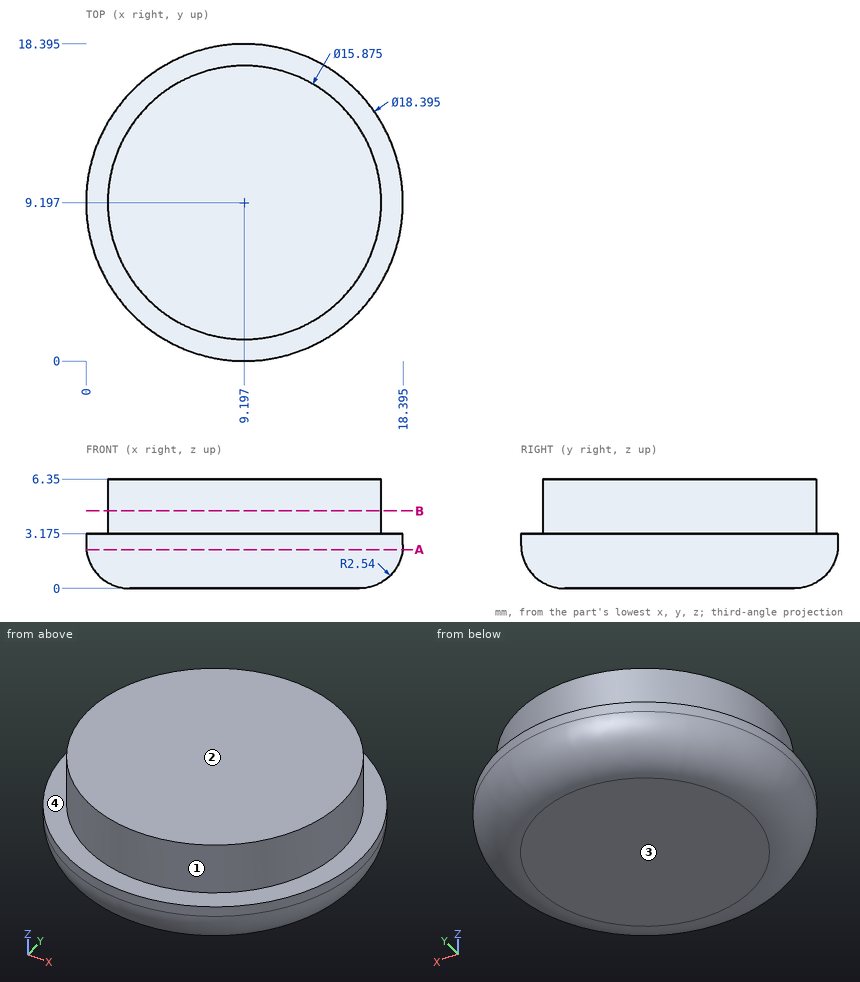
Answer from the drawing. Dimensions are ordinates in mm from the lowest x, y and z of the part. A direction names the side the tool comes from. Give positions to 0.01 mm unless a question says otherwise; leave off trailing zeros. Order: outer loops, then holes, each group sorted by start corner. A loop starts at its lowest first (then second) coordinate and runs counter-clockwise, first axis right, second up.
(1) Straight lines are drawn through the part: L1, parallel to Z at x = 3.5, y = 2.5 (1 decimal); L2, parallel to Y at x = 13.5, z = 3.25; L3, parallel to X at y = 4, z = 4.75 (1 decimal). For each, find the intervals that lie inside material, in ascending order.
(2) Find section B-B (z = 4.5). Give the vertices of the cut face in (x, y) (1 decimal), plus the area to 3 significant figures.
(3) For a pull along Y with two mould halves and no side action, classify the marked faces 1 and 2 as released by +Y, released by -Y, zero draft, split by the parting line, or undercut.
(4) Given pin 1 (3 mm diameter, centred on y = 7.5, z = 4.5, fed in from -X), flat-ended and moving along its own axis, determine where the tip first touches the part or whether it passes through.
(5) Find section A-A (z = 2.25). Give the vertices of the cut face in (x, y).
(6) For the marked faces 3 and 4, determine the directions among +Z, -Z, +X, -X, +Y, -Y from which every point of the face is accessible in a straight line to the end or side of a thin tool.
Result sheet:
1. L1: z = 1.2 to 3.2
1. L2: y = 2.53 to 15.87
1. L3: x = 3.2 to 15.2
2. outline: circle Ø15.9 at (9.2, 9.2)
2. area: 198 mm2
3. face 1: split by the parting line
3. face 2: zero draft
4. pin 1: stops at x = 0.05
5. outline: circle Ø18.36 at (9.2, 9.2)
6. face 3: -Z, +X, -X, +Y, -Y
6. face 4: +Z
